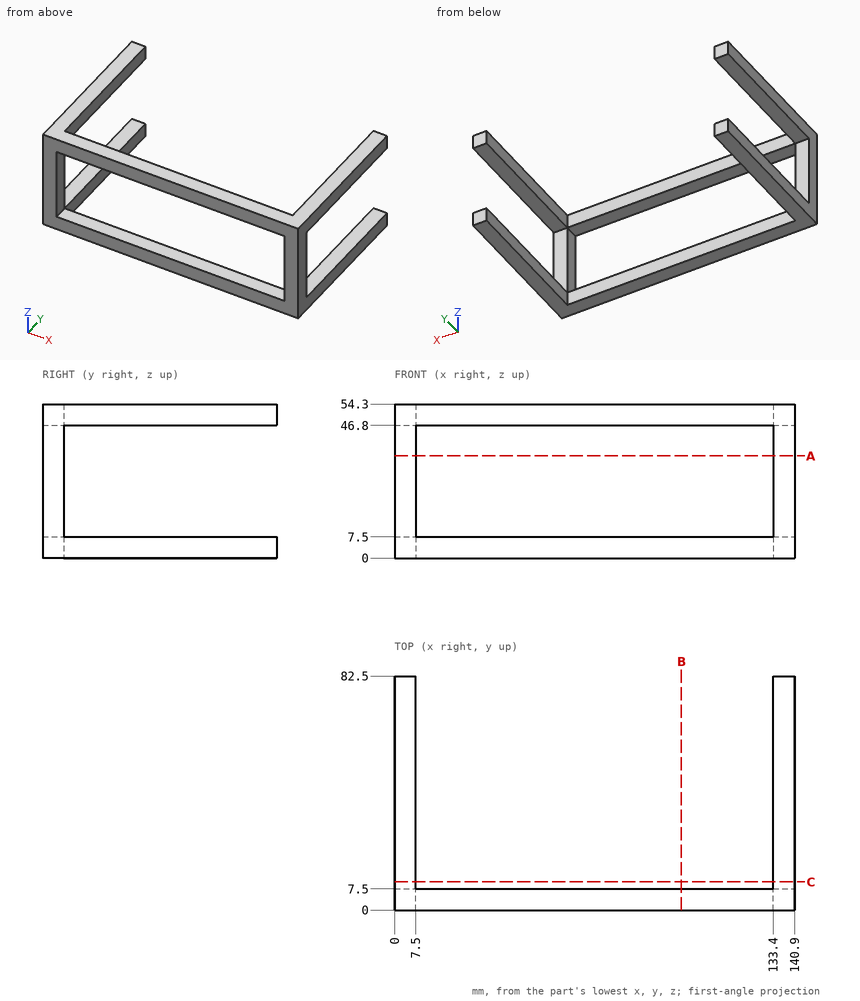
Could you check a few things on this drawing? It's one solid part, dimensions in mm from its lowest x, y, z. Coordinates: 2 decimals unless noted, no trailing zeros. Order: outer loops, then holes, each group sorted by start corner. A loop starts at its lowest first (then second) coordinate and runs counter-clockwise, first axis right, second up. Notation, with made-up numbers: M 49.25,-1 L 102.25,-1 A29 cw 102.25,29 Z; hole C 20.25,-1.75 d7. An arc over 180 degrees is marked long. Use one line per item in the form item = value. Start each with the question number.
1. Suppose I cut it at A-A on z = 36. Write out the boundary of the cut face in (x, y), then the cut area to 4 significant figures.
2. Please list where these lines run through material, in increasing order: line 1 (X direction, y = 32, z = 47.5); line 2 (Z direction, x = 6.5, y = 19.5); line 3 (Y direction, x = 10, z = 5.5).
3. For pin 1 (6 mm diameter, centred on x = 136.5, z = 29.5, fed in from +Y); pin 2 (8 mm diameter, centred on y = 38, z = 2.5, fed in from -X), each with a flat end and sliding along its axis, tell me the tip position at first contact or that it passes through.
4. Suppose I cut it at C-C on y = 10. Write out the boundary of the cut face in (x, z), then the cut area to 3 significant figures.
5. Suppose I cut it at B-B on x = 101. Write out the boundary of the cut face in (y, z), then the cut area to 4 significant figures.
Geometry says:
q1.outline = M 0,0 L 7.5,0 L 7.5,7.5 L 0,7.5 Z; M 133.4,0 L 140.9,0 L 140.9,7.5 L 133.4,7.5 Z
q1.area = 112.5 mm^2
q2.line_1 = 0 to 7.5, 133.4 to 140.9
q2.line_2 = 0 to 7.5, 46.8 to 54.3
q2.line_3 = 0 to 7.5
q3.pin_1 = 7.5
q3.pin_2 = 0
q4.outline = M 0,0 L 7.5,0 L 7.5,7.5 L 0,7.5 Z; M 0,46.8 L 7.5,46.8 L 7.5,54.3 L 0,54.3 Z; M 133.4,0 L 140.9,0 L 140.9,7.5 L 133.4,7.5 Z; M 133.4,46.8 L 140.9,46.8 L 140.9,54.3 L 133.4,54.3 Z
q4.area = 225 mm^2
q5.outline = M 0,0 L 7.5,0 L 7.5,7.5 L 0,7.5 Z; M 0,46.8 L 7.5,46.8 L 7.5,54.3 L 0,54.3 Z
q5.area = 112.5 mm^2
